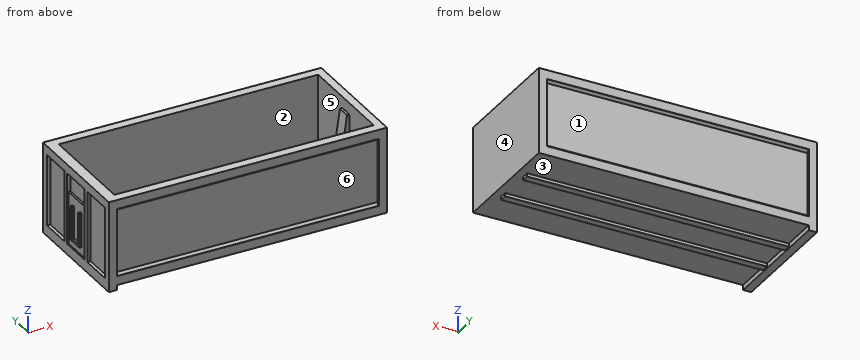
```python
from build123d import *

# Parameters (mm, degrees)
F1_DEPTH  = 32
F2_W      = 1
F2_H      = 10.5
F3_DEPTH  = 7.4
F4_W      = 7.4
F4_H      = 10.9
F5_DEPTH  = 1
F6_W      = 3.9333333333
F6_H      = 8.7
F6_W_2    = 1.9666666667
F7_DEPTH  = 0.4
F8_SIZE   = 0.3
F10_DEPTH = 0.8
F12_W     = 1
F12_H     = 14.8
F13_DEPTH = 0.2
F14_DEPTH = 0.3
F15_W     = 3.9333333333
F15_H     = 6.4
F16_DEPTH = 0.25
F18_DEPTH = 0.25


with BuildPart() as f1:
    # F0 (on Right) → F1 (new body)
    with BuildSketch(Plane.YZ):
        Polygon((-6.25, 10.9), (-7.4, 10.9), (-7.4, 9.8), (-7.05, 9.8), (-7.05, 1.5), (-7.4, 1.5), (-7.4, 0.4), (-2.9, 0.4), (-2.9, 0), (-2, 0), (-2, 0.4), (0, 0.4), (0, 1.2), (-6.25, 1.2), align=None)
    extrude(amount=F1_DEPTH)

    # F2 (on face) → F3 (join, through all)
    with BuildSketch(Plane.XZ.offset(7.4)):
        with Locations((32.5, 5.65)):
            Rectangle(F2_W, F2_H)
    extrude(amount=-F3_DEPTH)

    # F4 (on face) → F5 (join)
    with BuildSketch(Plane(origin=(0, 0, 0), x_dir=(0, -1, 0), z_dir=(-1, 0, 0))):
        with Locations((3.7, 5.45)):
            Rectangle(F4_W, F4_H)
    extrude(amount=F5_DEPTH)

    # F6 (on face) → F7 (cut)
    with BuildSketch(Plane(origin=(-1, 0, 0), x_dir=(0, -1, 0), z_dir=(-1, 0, 0))):
        with Locations((4.5333333333, 5.45)):
            Rectangle(F6_W, F6_H)
        with Locations((0.9833333333, 5.45)):
            Rectangle(F6_W_2, F6_H)
    extrude(amount=-F7_DEPTH, mode=Mode.SUBTRACT)

    # F8
    f8_edges = [f1.edges().sort_by_distance(p)[0] for p in [
        (16, -7.05, 1.5),
        (16, -7.05, 9.8),
    ]]
    chamfer(f8_edges, length=F8_SIZE)

    # F9 (on face) → F10 (join)
    with BuildSketch(Plane(origin=(0, 0, 0), x_dir=(-1, 0, 0), z_dir=(0, 1, 0))):
        Polygon((-32, 9.5), (-32, 1.2), (-30.5, 1.2), (-31.7, 9.5), align=None)
    extrude(amount=-F10_DEPTH)

    # F11: F1 across face


with BuildPart() as f1_1:
    add(f1.part)
    add(f1.part.mirror(Plane(origin=(19.2854383212, 0, 3.0068542852), x_dir=(-1, 0, 0), z_dir=(0, 1, 0))))

    # F12 (on face) → F13 (join)
    with BuildSketch(Plane(origin=(0, 0, 0), x_dir=(1, 0, 0), z_dir=(0, 0, -1))):
        with Locations((-0.5, 0)):
            Rectangle(F12_W, F12_H)
    extrude(amount=F13_DEPTH)

    # F14 (add): a face of the model
    f14_faces = [f1_1.faces().sort_by_distance(p)[0] for p in [
        (0, 0, 6.05),
    ]]
    extrude(f14_faces, amount=F14_DEPTH)

    # F15 (on face) → F16 (join)
    with BuildSketch(Plane(origin=(-0.6, 0, 0), x_dir=(0, -1, 0), z_dir=(-1, 0, 0))):
        with Locations((0, 4.3)):
            Rectangle(F15_W, F15_H)
    extrude(amount=F16_DEPTH)

    # F17 (on face) → F18 (join)
    with BuildSketch(Plane(origin=(-0.85, 0, 0), x_dir=(0, -1, 0), z_dir=(-1, 0, 0))):
        Polygon((-0.7, 6.3), (-1, 6.3), (-1, 2.1), (1, 2.1), (1, 6.3), (0.7, 6.3), (0.7, 2.4), (-0.7, 2.4), align=None)
    extrude(amount=F18_DEPTH)


solid = f1_1.part
```
Design review of the part built by this model. Coordinates are the model's own, in mm. Face numbers are marked on the shaded views. A direction names the side the tool comes from. Coordinates: 2 decimals unless noted, no trailing zeros. Order: outer loops, then holes, each group sorted by start corner. A loop starts at its lowest first (then second) coordinate and runs counter-clockwise, first axis right, second up.
1) Clearance check with flat-ended pins moving along their axes: pin 1 (5 mm diameter, centred on x = 23.5, y = 2, fed in from -Z); pin 2 (2 mm diameter, centred on x = 26, y = -4, fed in from -Z); pin 3 (6 mm diameter, centred on x = 11, y = -3, fed in from +Z); pin 4 (4.5 mm diameter, centred on y = 0, z = 4, fed in from -X). State where each tip first meets the part, or that it passes through.
2) Take a section at A-A, the plane y = 3.25. Give the boundary of the cut face in (x, z), and give its area (3 significant figures).
3) Wall thickness on line 1 along X through (y, z) = (0.25, 10); line 2 along Y through (x, z) = (31, 6.25); line 3 along X through (y, z) = (-1.25, 6): over which ranges is each line inside the solid? List them lowest first.
4) Take a section at D-D, the plane y = 0.25. Give the boundary of the cut face in (x, z).
5) Take a section at C-C, the plane x = 10. Give the boundary of the cut face in (y, z), and give its area (3 significant figures).
6) For the marked faces 1 and 2, list the 3-axis set-ups (+Z, -Z, +X, -X, +Y, -Y) from which the entire face can be reached by the end or side of a thin tool; tool diameter is ignored.
7) Mouldability with a two-part tool opening along Y and no side actions: class the marked faces 3, 4, 5 and 6 as +Y half, -Y half, draft (parallel to the pull), parting line (faces both ways), or undercut.
Returned:
1. pin 1: stops at z = 0
1. pin 2: stops at z = 0.4
1. pin 3: stops at z = 1.2
1. pin 4: stops at x = -1.1
2. outline: (-1, -0.2) - (0, -0.2) - (0, 0.4) - (33, 0.4) - (33, 10.9) - (32, 10.9) - (32, 1.2) - (0.3, 1.2) - (0.3, 10.9) - (-1, 10.9) - (-1, 9.8) - (-0.6, 9.8) - (-0.6, 1.1) - (-1, 1.1) - close
2. area: 46.6 mm2
3. line 1: x = -1 to 0.3, 32 to 33
3. line 2: y = -7.05 to -6.25, 6.25 to 7.05
3. line 3: x = -0.85 to 0.3, 32 to 33
4. outline: (-1.1, 2.1) - (-0.85, 2.1) - (-0.85, 1.1) - (-1, 1.1) - (-1, -0.2) - (0, -0.2) - (0, 0.4) - (33, 0.4) - (33, 10.9) - (32, 10.9) - (32, 9.5) - (31.7, 9.5) - (30.5, 1.2) - (0.3, 1.2) - (0.3, 10.9) - (-1, 10.9) - (-1, 9.8) - (-0.6, 9.8) - (-0.6, 7.5) - (-0.85, 7.5) - (-0.85, 2.4) - (-1.1, 2.4) - close
5. outline: (-7.4, 0.4) - (-2.9, 0.4) - (-2.9, 0) - (-2, 0) - (-2, 0.4) - (2, 0.4) - (2, 0) - (2.9, 0) - (2.9, 0.4) - (7.4, 0.4) - (7.4, 1.5) - (7.35, 1.5) - (7.05, 1.8) - (7.05, 9.5) - (7.35, 9.8) - (7.4, 9.8) - (7.4, 10.9) - (6.25, 10.9) - (6.25, 1.2) - (-6.25, 1.2) - (-6.25, 10.9) - (-7.4, 10.9) - (-7.4, 9.8) - (-7.35, 9.8) - (-7.05, 9.5) - (-7.05, 1.8) - (-7.35, 1.5) - (-7.4, 1.5) - close
5. area: 29.2 mm2
6. face 1: +Y
6. face 2: +Z
7. face 3: undercut
7. face 4: draft
7. face 5: undercut
7. face 6: -Y half
